Autodesk Inventor part; units mm, degrees
ref_plane "YZ Plane" through (0, 0, 0) normal (1, 0, 0) x (0, 1, 0)
ref_plane "XZ Plane" through (0, 0, 0) normal (0, 1, 0) x (-1, 0, 0)
ref_plane "XY Plane" through (0, 0, 0) normal (0, 0, 1) x (1, 0, 0)
sketch "Boceto1" plane through (0, 0, 0) normal (0, 1, 0) x (-1, 0, 0)
  line L0 (0, 0) -> (5.8, 0)
  line L1 (5.8, 0) -> (9.3, 0)
  line L2 (5.8, 0) -> (2.9, -5.0229)
  line L3 (2.9, -5.0229) -> (-2.9, -5.0229)
  line L4 (-2.9, -5.0229) -> (-5.8, 0)
  line L5 (-5.8, 0) -> (-2.9, 5.0229)
  line L6 (-2.9, 5.0229) -> (2.9, 5.0229)
  line L7 (2.9, 5.0229) -> (5.8, 0)
  line L8 (9.3, 0) -> (4.65, -8.054)
  line L9 (4.65, -8.054) -> (-4.65, -8.054)
  line L10 (-4.65, -8.054) -> (-9.3, 0)
  line L11 (-9.3, 0) -> (-4.65, 8.054)
  line L12 (-4.65, 8.054) -> (4.65, 8.054)
  line L13 (4.65, 8.054) -> (9.3, 0)
  dimension "d0" = 5.8
  dimension "d1" = 3.5
extrude "Extrusión1" add sketch "Boceto1" along normal blind 30
sketch "Boceto2" plane through (0, 30, 0) normal (0, 1, 0) x (1, 0, 0)
  line L0 (-4.65, 8.054) -> (-9.3, 0)
  line L1 (-9.3, 0) -> (-4.65, 8.054)
  line L2 (-4.65, 8.054) -> (4.65, 8.054)
  line L3 (4.65, 8.054) -> (9.3, 0)
  line L4 (9.3, 0) -> (4.65, -8.054)
  line L5 (4.65, -8.054) -> (-4.65, -8.054)
  line L6 (-4.65, -8.054) -> (-9.3, 0)
  point P0 (0, 0)
  point P1 (0, 0)
extrude "Extrusión2" add sketch "Boceto2" along normal blind 13.5 draft -12
sketch "Boceto3" plane through (0, 0, 0) normal (0, -1, 0) x (1, 0, 0)
  line L0 (9.3, 0) -> (5.9866, 0)
  line L1 (9.3, 0) -> (4.65, -8.054)
  line L2 (4.65, -8.054) -> (-4.65, -8.054)
  line L3 (-4.65, -8.054) -> (-9.3, 0)
  line L4 (-9.3, 0) -> (-4.65, 8.054)
  line L5 (-4.65, 8.054) -> (4.65, 8.054)
  line L6 (4.65, 8.054) -> (9.3, 0)
  point P0 (0, 0)
  point P1 (0, 0)
sketch "Boceto4" plane through (0, 0, 0) normal (0, -1, 0) x (1, 0, 0)
  line L0 (5.8, 0) -> (2.9, -5.0229)
  line L1 (2.9, -5.0229) -> (-2.9, -5.0229)
  line L2 (-2.9, -5.0229) -> (-5.8, 0)
  line L3 (-5.8, 0) -> (-2.9, 5.0229)
  line L4 (-2.9, 5.0229) -> (2.9, 5.0229)
  line L5 (2.9, 5.0229) -> (5.8, 0)
  point P0 (0, 0)
  point P1 (0, 0)
extrude "Extrusión3" add sketch "Boceto3" along normal blind 2
sketch "Boceto5" plane through (0, -2, 0) normal (0, -1, 0) x (1, 0, 0)
  line L0 (0, 0) -> (5.8, 0)
  line L1 (5.8, 0) -> (2.9, -5.0229)
  line L2 (2.9, -5.0229) -> (-2.9, -5.0229)
  line L3 (-2.9, -5.0229) -> (-5.8, 0)
  line L4 (-5.8, 0) -> (-2.9, 5.0229)
  line L5 (-2.9, 5.0229) -> (2.9, 5.0229)
  line L6 (2.9, 5.0229) -> (5.8, 0)
  dimension "d8" = 5.8
extrude "Extrusión4" cut sketch "Boceto5" against normal blind 2
sketch "Boceto6" plane through (0, 43.5, 0) normal (0, 1, 0) x (1, 0, 0)
  line L0 (-1.75, 0) -> (-1.75, 2.1213)
  line L1 (-1.75, 0) -> (-1.75, -2.1213)
  line L2 (1.75, 0) -> (1.75, 2.1213)
  line L3 (1.75, 0) -> (1.75, -2.1213)
  arc A0 (-1.75, -2.1213) -> (1.75, -2.1213) centre (0, 0) ccw
  arc A1 (1.75, 2.1213) -> (-1.75, 2.1213) centre (0, 0) ccw
extrude "Extrusión5" cut sketch "Boceto6" against normal blind 5.5
sketch "Boceto8" plane through (-9.3, -2, 0) normal (-0.8660254, 0, -0.5) x (-0.5, 0, 0.8660254)
  line L0 (-4.65, 11) -> (-2.65, 11)
  line L1 (-4.65, 11) -> (-6.65, 11)
  line L2 (-6.65, 21) -> (-2.65, 21)
  line L3 (-2.65, 21) -> (-2.65, 11)
  line L4 (-6.65, 11) -> (-6.65, 21)
extrude "Extrusión7" add sketch "Boceto8" along normal blind 5
fillet "Empalme2" radius 1.5 2 edges at (-12.3051, 14, -4.795) (-10.3051, 14, -8.2591)
sketch "Boceto9" plane through (4.075, -2, 8.054) normal (0, 0, 1) x (1, 0, 0)
  line L0 (0, 0) -> (0, 32)
  line L1 (0, 0) -> (0, 16)
  line L2 (-1.75, 32) -> (1.15, 32)
  line L3 (-9.3, 32) -> (-9.3, 0)
  line L4 (-4.65, 11) -> (-6.65, 11)
  line L5 (-6.65, 11) -> (-2.65, 11)
  line L6 (-2.65, 11) -> (-2.65, 21)
  line L7 (-2.65, 21) -> (-4.65, 21)
  line L8 (-4.65, 21) -> (-6.65, 21)
  line L9 (-6.65, 21) -> (-6.65, 11)
  point P0 (-4.65, 2)
extrude "Extrusión8" add sketch "Boceto9" along normal blind 5
sketch "Boceto10" plane through (4.9375, -2, -7.5561) normal (0.8660254, 0, -0.5) x (-0.5, 0, -0.8660254)
  line L0 (0, 0) -> (0, 32)
  line L1 (0, 0) -> (0, 16)
  line L2 (-1.75, 32) -> (1.15, 32)
  line L3 (-9.3, 32) -> (-9.3, 0)
  line L4 (-4.65, 11) -> (-6.65, 11)
  line L5 (-6.65, 11) -> (-2.65, 11)
  line L6 (-2.65, 11) -> (-2.65, 21)
  line L7 (-2.65, 21) -> (-4.65, 21)
  line L8 (-4.65, 21) -> (-6.65, 21)
  line L9 (-6.65, 21) -> (-6.65, 11)
  point P0 (-4.65, 2)
extrude "Extrusión9" add sketch "Boceto10" along normal blind 5
fillet "Empalme3" radius 1.5 4 edges at (-2.575, 14, 13.054) (1.425, 14, 13.054) (12.5926, 14, -4.297) (10.5926, 14, -7.7611)
properties part number "acopladorV4"
Design review of the part built by this model. Coordinates are the model's own, in mm. A direction names the side the tool comes from. Give positions to 0.01 mm unless a question says otherwise; leave off trailing zeros. Loops run counter-clockwise (first coordinate to the right, second up) from the corner with the lowest first, then second, coordinate; pieces in that order, holes last. Notation, with made-up numbers: M -40,-11.75 L 16,-11.75 A19 ccw 16,10.25 Z; hole C -6.5,75.5 d2. An arc over 180 degrees is marked long. Write item = value, one per line.
Q1. Draft analysis for pull direction X (two halves, no side actions). For faces 1 (the flat face through (0, 14, -8.054)), 2 (the flat face through (4.33, 13.78, 2.55)), 3 (the cylindrical face through (11.997, 13.93, -4.474)), 4 (the flat face through (0, 14, -5.023)), state which applies: +X half, -X half, draft (parallel to the pull), parting line (faces both ways), or undercut.
Output values:
face_1 = draft
face_2 = undercut
face_3 = +X half
face_4 = undercut
Q2. We need section C-C (z = 9). Give the boundary of the cut face in (x, y) (3 decimals).
Output values:
outline = M -2.575,9 L 1.425,9 L 1.425,19 L -2.575,19 Z
Q3. We need section B-B (x = 0.75). Give the boundary of the cut face in (y, z), plus the area to 3 significant figures.
Output values:
outline = M -2,-8.05 L 30,-8.05 L 43.5,-5.18 L 43.5,-2.65 L 38,-2.65 L 38,2.65 L 43.5,2.65 L 43.5,5.18 L 30,8.05 L 19,8.05 L 19,12.81 L 9,12.81 L 9,8.05 L -2,8.05 L -2,5.02 L 30,5.02 L 30,-5.02 L -2,-5.02 Z
area = 391 mm^2
Q4. To check wall thickness, follow line 1 (Z direction, x = 1.5, y = 24); line 2 (X direction, y = 28.5, z = -2); line 3 (Y direction, x = -4.25, z = -1). State the ranges of each line that lie inside material, in increasing order. Write a range as [from, to].
Output values:
line_1 = [-8.05, -5.02], [5.02, 8.05]
line_2 = [-8.15, -4.65], [4.65, 8.15]
line_3 = [30, 43.5]
Q5. Insertion check: pin 1 (1 mm diameter, centred on x = 4.5, y = 28, fed in from +Z); pin 2 (5 mm diameter, centred on y = 8.5, z = 5, fed in from +X); pin 3 (2.5 mm diameter, centred on x = 10, z = -5.5, fed in from +Y). Each pin has a flat end and moves straight along its axis. Give the tip position at first contact, or say it passes through.
Output values:
pin_1 = 8.05
pin_2 = 7.86
pin_3 = 19
Q6. We need section A-A (y = 6.5). Give the boundary of the cut face in (x, z), plus the area to 3 significant figures.
Output values:
outline = M -9.3,0 L -4.65,-8.05 L 4.65,-8.05 L 9.3,0 L 4.65,8.05 L -4.65,8.05 Z; hole M -5.8,0 L -2.9,-5.02 L 2.9,-5.02 L 5.8,0 L 2.9,5.02 L -2.9,5.02 Z
area = 137 mm^2
Q7. For faces 5 (the flat face through (7.757, 13.93, -6.124)), 6 (the cylindrical face through (-0.03, 40.79, 2.75)), 7 (the flat face through (-4.33, 13.78, -2.55)), list the 3-axis set-ups (+Z, -Z, +X, -X, +Y, -Y) from which the entire face can be reached by the end or side of a thin tool; tool diameter is ignored.
Output values:
face_5 = -Z, +Y, -Y
face_6 = +Y
face_7 = -Y
